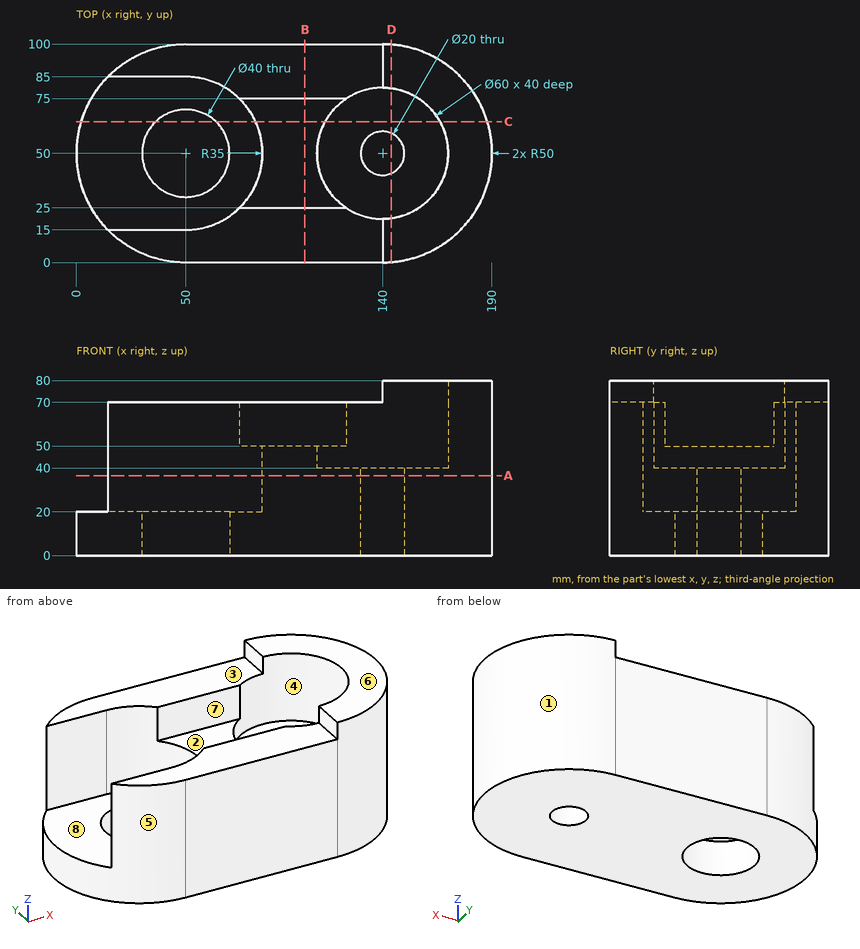
The figure shows three views and two pictorial views of one solid part (mm, origin at its lowest corner). Answer the questions. A direction names the side the tool comes from. Give positions to 0.01 mm unless a question says otherwise; leave off trailing zeros. Write each loop counter-clockwise with the first axis right and the second up, starting at its lowest first coordinate (ties: lowest second). Pieces come first, ordered by that corner, then holes. Notation, with made-up numbers: (-37, 66.25) -> (-30, 66.25) arc R16 cw to (-30, 70.25) -> close; hole circle Ø3 at (29, -31.75). An arc over 180 degrees is marked (long way). Use one line per item in the form item = value.
1) Section D-D on x = 144 is taken. Write down the section's boundary in (y, z), plus the area to 3 significant figures.
Result:
outline = (0.16, 0) -> (40.83, 0) -> (40.83, 40) -> (20.27, 40) -> (20.27, 80) -> (0.16, 80) -> close; (59.17, 0) -> (99.84, 0) -> (99.84, 80) -> (79.73, 80) -> (79.73, 40) -> (59.17, 40) -> close
area = 4,860 mm²
2) Section B-B on x = 104.5 is taken. Write down the section's boundary in (y, z).
Result:
outline = (0, 0) -> (100, 0) -> (100, 70) -> (75, 70) -> (75, 50) -> (25, 50) -> (25, 70) -> (0, 70) -> close
3) Section C-C on y = 64.5 is taken. Write down the section's boundary in (x, z).
Result:
outline = (2.15, 0) -> (36.23, 0) -> (36.23, 20) -> (2.15, 20) -> close; (63.77, 0) -> (187.85, 0) -> (187.85, 80) -> (166.26, 80) -> (166.26, 40) -> (113.74, 40) -> (113.74, 50) -> (81.86, 50) -> (81.86, 20) -> (63.77, 20) -> close
4) For a pull along Y with two mould halves and no side action, classify the marked faces 5, 6, 7 and 8 as +Y half, -Y half, draft (parallel to the pull), parting line (faces both ways), or undercut.
Result:
face_5 = parting line
face_6 = draft
face_7 = undercut
face_8 = undercut
5) Section A-A on z = 36.5 is taken. Write down the section's boundary in (x, y), plus the area to 3 significant figures.
Result:
outline = (14.29, 15) arc R50 ccw to (50, 0) -> (140, 0) arc R50 ccw to (140, 100) -> (50, 100) arc R50 ccw to (14.29, 85) -> (50, 85) arc R35 cw to (50, 15) -> close; hole circle Ø20 at (140, 50)
area = 11,400 mm²
6) Each of these flat-tipped pins is pushed along its axis until it touches: P1, Ø2, axis at y = 44.5, z = 65, coming from the -X side; P2, Ø6, axis at y = 48, z = 69.5, coming from the +X side; P3, Ø6, axis at x = 97.5, y = 89, coming from the -Z side; P4, Ø5, axis at y = 88, z = 74, coming from the -X side. Where does it stop, or does it pass through?
Result:
P1 = 169.29
P2 = 190
P3 = 0
P4 = 140
7) A tool of negligible diameter and unlimited length cuts with its end or side. For the marked faces 1, 2, 3 and 4, from which of +Z, -Z, +X, -X, +Y, -Y can it reach the whole face along a straight path? Write none if from no direction.
Result:
face_1 = +Z, -Z, +X
face_2 = +Z, -X
face_3 = +Z, -X, +Y, -Y
face_4 = +Z
8) Straight lines are drawn through the part: probe 1 along Y at (x, z) = (140, 28); probe 2 along Y at (x, z) = (50, 35.5); probe 3 along Z at (x, y) = (68, 88.5). For each, find the intervals that lie inside material, in ascending order.
Result:
probe_1 = 0 to 40, 60 to 100
probe_2 = 0 to 15, 85 to 100
probe_3 = 0 to 70
